from build123d import *

# Parameters (mm, degrees)
F0_R     = 10
F0_R_2   = 20
F1_DEPTH = 25


with BuildPart() as f1:
    # F0 (on Top) → F1 (new body)
    with BuildSketch(Plane.XY):
        Polygon((72.579548, 39.166598), (-51.420452, 39.166598), (-51.420452, -25.833402), (-51.420452, -43.833402), (-21.420452, -43.833402), (25.579548, -43.833402), (25.579548, -63.833402), (49.079548, -63.833402), (72.579548, -63.833402), (72.579548, 25.166598), align=None)
        with Locations((-21.420452, -25.833402)):
            Circle(F0_R, mode=Mode.SUBTRACT)
        with Locations((48.579548, -30.833402)):
            Circle(F0_R_2, mode=Mode.SUBTRACT)
        with BuildLine():
            Line((-3.420452, 28.166598), (59.579548, 28.166598))
            ThreePointArc((59.579548, 28.166598), (65.236402, 25.823453), (67.579548, 20.166598))
            ThreePointArc((67.579548, 20.166598), (65.236402, 14.509744), (59.579548, 12.166598))
            Line((59.579548, 12.166598), (-3.420452, 12.166598))
            ThreePointArc((-3.420452, 12.166598), (-9.077307, 14.509744), (-11.420452, 20.166598))
            ThreePointArc((-11.420452, 20.166598), (-9.077307, 25.823453), (-3.420452, 28.166598))
        make_face(mode=Mode.SUBTRACT)
    extrude(amount=F1_DEPTH)


solid = f1.part
Could you check a few things on this model? Use its own coordinates, in mm. A direction names the side the tool comes from. Round coordinates to 2 decimals unless told otherwise and drop trailing zeros. Write each loop counter-clockwise with the first axis right and the second up, starting at its lowest first coordinate (ties: lowest second). Pieces come first, ordered by that corner, then holes. Notation, with made-up numbers: (36, 84) -> (54, 84) arc R27 ccw to (54, 121) -> close; hole circle Ø5 at (-21.75, 39.5). An arc over 180 degrees is marked (long way). Use a Markdown table: item, result.
1. If we section it at D-D (z = 2.25): List the corners of the cut face in (x, y) for me, then the cut area to 3 significant figures.
Answer key:
| item | result |
|---|---|
| outline | (-51.42, -43.83) -> (25.58, -43.83) -> (25.58, -63.83) -> (72.58, -63.83) -> (72.58, 39.17) -> (-51.42, 39.17) -> close; hole circle Ø20 at (-21.42, -25.83); hole (-11.42, 20.17) arc R8 ccw to (-3.42, 12.17) -> (59.58, 12.17) arc R8 ccw to (67.58, 20.17) arc R8 ccw to (59.58, 28.17) -> (-3.42, 28.17) arc R8 ccw to start; hole circle Ø40 at (48.58, -30.83) |
| area | 8,450 mm^2 |
2. If we section it at B-B (y = -34.5): List the corners of the cut face in (x, z) for me.
Answer key:
| item | result |
|---|---|
| outline | (-51.42, 0) -> (-26.41, 0) -> (-26.41, 25) -> (-51.42, 25) -> close; (-16.43, 0) -> (28.92, 0) -> (28.92, 25) -> (-16.43, 25) -> close; (68.24, 0) -> (72.58, 0) -> (72.58, 25) -> (68.24, 25) -> close |
3. We'd pull the mould along Y, two halves only. Please class faces 4 (the face through (72.58, -13, 12)), 5 (the face through (28, 28.167, 12)), 6 (the face through (-13, -43.833, 12)): +Y half, -Y half, draft (parallel to the pull), parting line (faces both ways), or undercut.
Answer key:
| item | result |
|---|---|
| face 4 | draft |
| face 5 | undercut |
| face 6 | -Y half |
4. Please list where these lines run through material, in increasing order: probe 1 along Y at (x, z) = (8, 15.75); probe 2 along X at (y, z) = (-19, 4.5); probe 3 along X at (y, z) = (-33, 1.75).
Answer key:
| item | result |
|---|---|
| probe 1 | y = -43.83 to 12.17, 28.17 to 39.17 |
| probe 2 | x = -51.42 to -28.72, -14.12 to 32.46, 64.7 to 72.58 |
| probe 3 | x = -51.42 to -28.39, -14.45 to 28.7, 68.46 to 72.58 |
5. If we section it at A-A (x = 12.5): List the corners of the cut face in (y, z) for me, then the cut area to 4 significant figures.
Answer key:
| item | result |
|---|---|
| outline | (-43.83, 0) -> (12.17, 0) -> (12.17, 25) -> (-43.83, 25) -> close; (28.17, 0) -> (39.17, 0) -> (39.17, 25) -> (28.17, 25) -> close |
| area | 1,675 mm^2 |
6. For pin 1 Ø6 at (y, z) = (-57, 16.5) entering from -X; pin 2 Ø4 at (x, y) = (16, 15) entering from +Z; pin 3 Ø7.5 at (x, z) = (-5, 9.5) entering from -Y, each with a flat end and sliding along its axis, tell me the tip position at first contact or that it passes through.
Answer key:
| item | result |
|---|---|
| pin 1 | stops at x = 25.58 |
| pin 2 | passes through |
| pin 3 | stops at y = -43.83 |
7. If we section it at C-C (y = -48.5): List the corners of the cut face in (x, z) for me.
Answer key:
| item | result |
|---|---|
| outline | (25.58, 0) -> (39.2, 0) -> (39.2, 25) -> (25.58, 25) -> close; (57.95, 0) -> (72.58, 0) -> (72.58, 25) -> (57.95, 25) -> close |
8. Which directions (+Z, -Z, +X, -X, +Y, -Y) give clear straight access to the entire face, cutting with the end or side of a thin tool? Please do faces 1 (the face through (25.58, -54, 12)), 2 (the face through (10, 0, 0)), 3 (the face through (29, 12.167, 12)).
Answer key:
| item | result |
|---|---|
| face 1 | +Z, -Z, -X, -Y |
| face 2 | -Z, +X, -X, +Y, -Y |
| face 3 | +Z, -Z |
